Can you work these out from the model? Positions are in its coordinate system, mm. A direction names the side the tool comes from. Coordinates: 2 decimals unless noted, no trailing zeros. Order: outer loops, then holes, each group sorted by start corner. A loop starts at its lowest first (then second) coordinate and runs counter-clockwise, first axis right, second up. Notation, with made-up numbers: (-11.5, 15) - (13.5, 15) arc R15 ccw to (13.5, 38) - close; hole circle Ø11 at (10, 65.25). An arc over 180 degrees is marked (long way). Return JSON: item names as keys, results as strings. Group by question number.
1) If we mould it in two halves opening along X, with no side actions, what happens to faces 5 (the face through (25, -25, -10)), 6 (the face through (-0.086, -6, 0)), 7 (the face through (44.914, -4, 0))? For each: pulls with the +X half, pulls with the -X half, needs draft (parallel to the pull), parting line crosses it, or undercut.
2) Imagine slicing it at A-A (y = -18.5). Write out the boundary of the cut face in (x, z).
3) For pin 1 Ø6.5 at (x, z) = (17.5, 8) entering from +Y; pin 2 Ø0.9 at (x, y) = (34.5, 14.5) entering from -Z; pin 3 Ø1 at (x, z) = (6.5, -3.5) entering from +Y, each with a flat end and sliding along its axis, tell me the tip position at first contact or that it passes through.
4) Imagine slicing it at C-C (z = 8.25). Write out the boundary of the cut face in (x, y), and give its area (3 significant figures).
5) Which directions (+Z, -Z, +X, -X, +Y, -Y) give clear straight access to the entire face, cutting with the end or side of a thin tool? Please do faces 1 (the face through (7, -4, -4)), 2 (the face through (25, -23.86, 7)), 3 (the face through (25, -20.86, 3)), 4 (the face through (42, -20.86, -3)).
6) If I drill on line 1 along X through (y, z) = (-8, 7.25); line 2 along X through (y, z) = (13, -3.75); line 3 along Y through (x, z) = (17, 2.25), over which ranges is the centre line in solid material (lowest first)?
7) Imagine slicing it at D-D (y = -23). Write out the boundary of the cut face in (x, z), and give its area (3 significant figures).
8) Imagine slicing it at B-B (x = 39). Write out the boundary of the cut face in (y, z), and give its area (3 significant figures).
Autodesk Inventor part; units mm, degrees
ref_plane "YZ Plane" through (0, 0, 0) normal (1, 0, 0) x (0, 1, 0)
ref_plane "XZ Plane" through (0, 0, 0) normal (0, 1, 0) x (-1, 0, 0)
ref_plane "XY Plane" through (0, 0, 0) normal (0, 0, 1) x (1, 0, 0)
sketch "Sketch1" plane through (0, 0, 0) normal (0, 0, 1) x (1, 0, 0)
  line L0 (4.914, 16.1404) -> (44.914, 16.1404)
  line L1 (44.914, 16.1404) -> (44.914, -23.8596)
  line L2 (44.914, -23.8596) -> (4.914, -23.8596)
  line L3 (4.914, -23.8596) -> (4.914, 16.1404)
  line L4 (49.914, 21.1404) -> (-0.086, 21.1404)
  line L5 (-0.086, 21.1404) -> (-0.086, -28.8596)
  line L6 (-0.086, -28.8596) -> (49.914, -28.8596)
  line L7 (49.914, -28.8596) -> (49.914, 21.1404)
  line L8 (4.914, 16.1404) -> (-0.086, 16.1404)
  line L9 (44.914, 16.1404) -> (49.914, 16.1404)
  line L10 (4.914, -20.8596) -> (44.914, -20.8596)
  line L11 (4.914, 13.1404) -> (44.914, 13.1404)
  line L12 (9.914, 13.1404) -> (9.914, -20.8596)
  line L13 (39.914, 13.1404) -> (39.914, -20.8596)
  point P0 (0, 0)
  dimension "d0" = 40
  dimension "d1" = 40
  dimension "d2" = 5
  dimension "d3" = 3
  dimension "d4" = 3
  dimension "d5" = 5
  dimension "d6" = 5
extrude "Extrusion1" add sketch "Sketch1" along normal mid plane 20 contours L3 L2 L1 L9 L7 L6 L5 L8
extrude "Extrusion2" add sketch "Sketch1" along normal blind 4 contours L0 L1 L11 L3 | L10 L1 L2 L3
extrude "Extrusion3" cut sketch "Sketch1" along normal blind 2 contours L0 L1 L11 L3 | L10 L1 L2 L3
extrude "Extrusion4" add sketch "Sketch1" against normal blind 4 contours L11 L12 L10 L3 | L1 L10 L13 L11
extrude "Extrusion5" cut sketch "Sketch1" against normal blind 2 contours L11 L12 L10 L3 | L1 L10 L13 L11
properties part number "Sensorroom"
Calculated:
{
 "1": {"face 5": "needs draft", "face 6": "pulls with the -X half", "face 7": "undercut"},
 "2": {"outline": "(-0.09, -10) - (4.91, -10) - (4.91, -4) - (9.91, -4) - (9.91, -2) - (4.91, -2) - (4.91, 10) - (-0.09, 10) - close; (39.91, -4) - (44.91, -4) - (44.91, -10) - (49.91, -10) - (49.91, 10) - (44.91, 10) - (44.91, -2) - (39.91, -2) - close"},
 "3": {"pin 1": "y = -23.86", "pin 2": "z = 2", "pin 3": "y = 13.14"},
 "4": {"outline": "(-0.09, -28.86) - (49.91, -28.86) - (49.91, 16.14) - (44.91, 16.14) - (44.91, -23.86) - (4.91, -23.86) - (4.91, 16.14) - (-0.09, 16.14) - close", "area": "650 mm2"},
 "5": {"face 1": "-Z, +Y", "face 2": "+Z, +Y", "face 3": "+Z", "face 4": "-Z"},
 "6": {"line 1": "-0.09 to 4.91, 44.91 to 49.91", "line 2": "-0.09 to 9.91, 39.91 to 49.91", "line 3": "-28.86 to -20.86, 13.14 to 16.14"},
 "7": {"outline": "(-0.09, -10) - (4.91, -10) - (4.91, 2) - (44.91, 2) - (44.91, -10) - (49.91, -10) - (49.91, 10) - (44.91, 10) - (44.91, 4) - (4.91, 4) - (4.91, 10) - (-0.09, 10) - close", "area": "280 mm2"},
 "8": {"outline": "(-28.86, -10) - (-23.86, -10) - (-23.86, 2) - (-20.86, 2) - (-20.86, 4) - (-23.86, 4) - (-23.86, 10) - (-28.86, 10) - close; (13.14, 2) - (16.14, 2) - (16.14, 4) - (13.14, 4) - close", "area": "112 mm2"}
}
